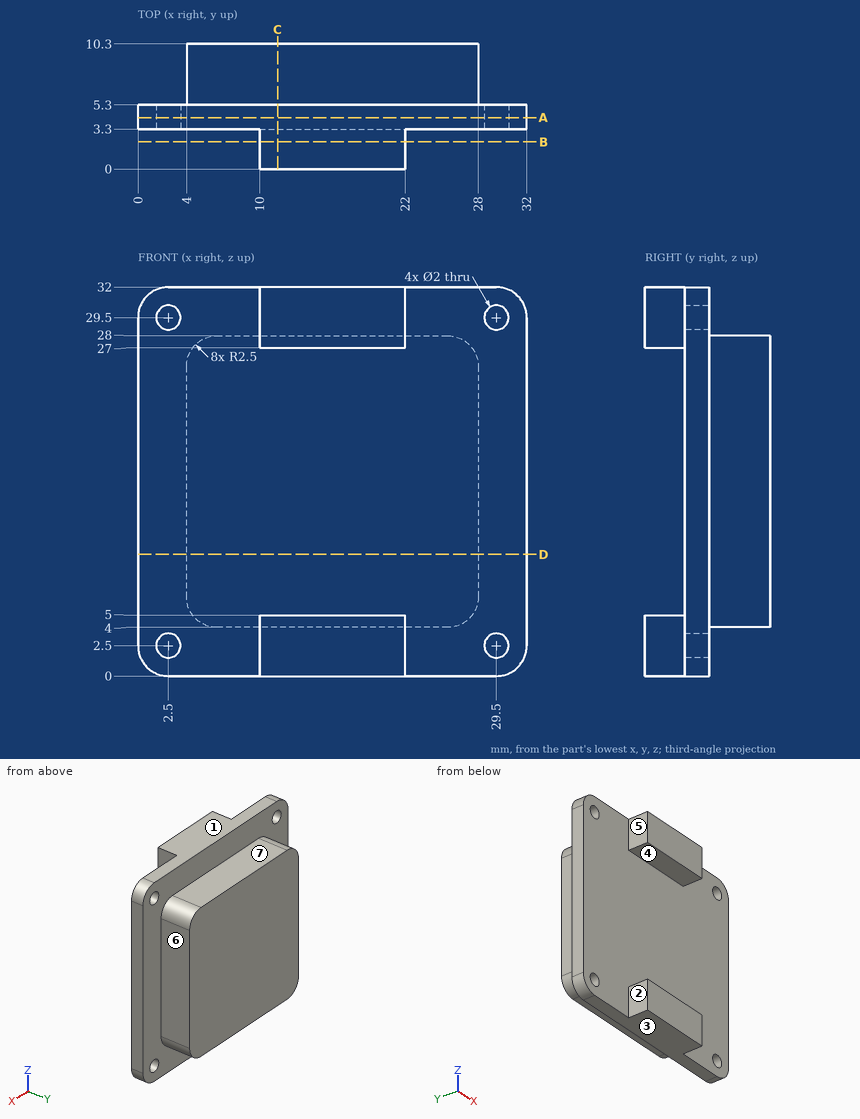
Part print with two shaded views. Sizes in mm from the minimum x, y, z corner. A direction names the side the tool comes from. Coordinates: 2 decimals unless noted, no trailing zeros. Order: outer loops, then holes, each group sorted by start corner. A loop starts at its lowest first (then second) coordinate and runs counter-clockwise, first axis right, second up. Notation, with made-up numbers: M 87.5,80.5 L 116.5,80.5 A33 ccw 116.5,110.5 Z; hole C -4,64 d6. An arc over 180 degrees is marked long. One line per question, with ' | ' between items. Start each with the question number.
1. Mould opens along Z. For the marked faces 1, 2, 3 and 4 say: +Z half, -Z half, draft (parallel to the pull), parting line (faces both ways), or undercut.
2. Cut at D-D (z = 10). Write the cut outline in (x, y).
3. Flat gauge pins, fed straight in: P1, Ø2.5, axis at x = 13, y = 8.5, coming from the -Z side; P2, Ø3.5, axis at y = 1, z = 2.5, coming from the -X side; P3, Ø3.5, axis at x = 16.5, y = 1.5, coming from the -Z side; P4, Ø2.5, axis at x = 2.5, z = 29.5, coming from the +Y side. Where does each tip first touch, or does it go through?
4. Tool access for the marked faces 5, 6 and 7: list every direction of +Z, -Z, +X, -X, +Y, -Y with a clear straight run to the whole face (end or side of a thin tool).
5. Cut at C-C (x = 11.5). Write the cut outline in (y, z), plus the area to 3 significant figures.
6. Wall check: line 1 along Z through (x, y) = (29.5, 4.6); line 2 along Z through (x, y) = (11.5, 1.75). Give the ranges that are in metal, low to high. Write a range as [from, to].
7. Cut at A-A (y = 4.25). Write the cut outline in (x, z).
8. Cut at B-B (y = 2.25). Write the cut outline in (x, z), plus the area to 3 significant figures.
The answers:
1) face 1: +Z half | face 2: draft | face 3: -Z half | face 4: undercut
2) outline: M 0,3.3 L 32,3.3 L 32,5.3 L 28,5.3 L 28,10.3 L 4,10.3 L 4,5.3 L 0,5.3 Z
3) P1: stops at z = 4 | P2: stops at x = 10 | P3: stops at z = 0 | P4: stops at y = 5.3
4) face 5: +Z, -Z, -X, -Y | face 6: +Z, -Z, +X, +Y | face 7: +Z, +X, -X, +Y
5) outline: M 0,0 L 5.3,0 L 5.3,4 L 10.3,4 L 10.3,28 L 5.3,28 L 5.3,32 L 0,32 L 0,27 L 3.3,27 L 3.3,5 L 0,5 Z | area: 217 mm2
6) line 1: z = [0, 1.5], [3.5, 28.5], [30.5, 32] | line 2: z = [0, 5], [27, 32]
7) outline: M 0,2.5 A2.5 ccw 2.5,0 L 29.5,0 A2.5 ccw 32,2.5 L 32,29.5 A2.5 ccw 29.5,32 L 2.5,32 A2.5 ccw 0,29.5 Z; hole C 2.5,2.5 d2; hole C 2.5,29.5 d2; hole C 29.5,2.5 d2; hole C 29.5,29.5 d2
8) outline: M 10,0 L 22,0 L 22,5 L 10,5 Z; M 10,27 L 22,27 L 22,32 L 10,32 Z | area: 120 mm2
